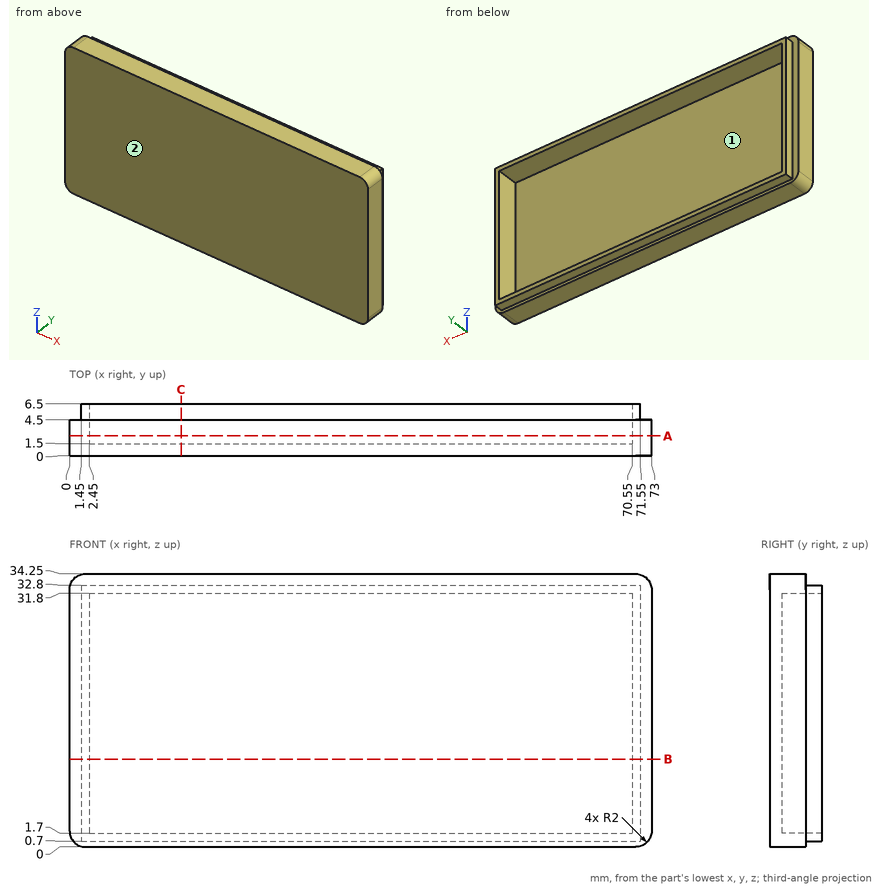
Geometry check sheet. Reference: drawing and pictorial views, mm from the part's lowest x, y, z. Coordinates: 2 decimals unless noted, no trailing zeros. Write each loop counter-clockwise with the first axis right and the second up, starting at its lowest first coordinate (ties: lowest second). Pieces come first, ordered by that corner, then holes. Notation, with made-up numbers: (77.5, -24) -> (96.5, -24) arc R24 cw to (96.5, -13) -> close; hole circle Ø3 at (84, -30.5). An arc over 180 degrees is marked (long way). One line per question, with ' | ' between items.
1. Cross-section at C-C on x = 14. Record the cut outline in (y, z), and give its area (3 significant figures).
Answers:
outline: (0, 0) -> (4.5, 0) -> (4.5, 0.7) -> (6.5, 0.7) -> (6.5, 1.7) -> (1.5, 1.7) -> (1.5, 31.8) -> (6.5, 31.8) -> (6.5, 32.8) -> (4.5, 32.8) -> (4.5, 34.25) -> (0, 34.25) -> close | area: 67.8 mm²
2. Cross-section at B-B on z = 11. Record the cut outline in (x, y), and give its area (3 significant figures).
Answers:
outline: (0, 0) -> (73, 0) -> (73, 4.5) -> (71.55, 4.5) -> (71.55, 6.5) -> (70.55, 6.5) -> (70.55, 1.5) -> (2.45, 1.5) -> (2.45, 6.5) -> (1.45, 6.5) -> (1.45, 4.5) -> (0, 4.5) -> close | area: 128 mm²
3. Cross-section at A-A on y = 2.5. Record the cut outline in (x, z), and give its area (3 significant figures).
Answers:
outline: (0, 2) arc R2 ccw to (2, 0) -> (71, 0) arc R2 ccw to (73, 2) -> (73, 32.25) arc R2 ccw to (71, 34.25) -> (2, 34.25) arc R2 ccw to (0, 32.25) -> close; hole (2.45, 1.7) -> (70.55, 1.7) -> (70.55, 31.8) -> (2.45, 31.8) -> close | area: 447 mm²
4. Draft check along Z on the marked faces 1 and 2. Enter one of: +Z half, -Z half, draft (parallel to the pull), parting line (faces both ways), or undercut.
Answers:
face 1: undercut | face 2: draft
5. Depth check by flat-ended pin: pin 1 Ø1 at (x, z) = (42, 9) entering from +Y; pin 2 Ø1 at (y, z) = (5.5, 13) entering from +X; pin 3 Ø0.6 at (y, z) = (5.5, 13) entering from -X. Enter the tip coordinate at first touch or a pass-through.
Answers:
pin 1: stops at y = 1.5 | pin 2: stops at x = 71.55 | pin 3: stops at x = 1.45
6. Thickness scan on probe 1 along Z at (x, y) = (51, 3.25); probe 2 along X at (y, z) = (6, 15.5); probe 3 along Z at (x, y) = (56, 5). Record the ranges inside material, lowest first. Write a range as from..to.
Answers:
probe 1: z = 0..1.7, 31.8..34.25 | probe 2: x = 1.45..2.45, 70.55..71.55 | probe 3: z = 0.7..1.7, 31.8..32.8
